For this review, take the finished solid that the model builds, in its own axes (mm). Face numbers are marked on the shaded views. A direction names the side the tool comes from. Round coordinates to 2 decimals unless told otherwise and drop trailing zeros. Write each loop counter-clockwise with the first axis right and the second up, starting at its lowest first coordinate (ties: lowest second). Pieces come first, ordered by that corner, then holes. Notation, with made-up numbers: (78, 83.25) -> (126, 83.25) arc R14 cw to (126, 103.25) -> close; hole circle Ø7 at (29, -8). An arc over 180 degrees is marked (long way). Answer in a Markdown table with one row per item. Add a question column.
```python
from build123d import *

# Parameters (mm, degrees)
SKETCH1_R           = 1.425
BOSS_EXTRUDE1_DEPTH = 4
SKETCH2_W           = 217.15
SKETCH2_H           = 5
BOSS_EXTRUDE2_DEPTH = 24
FILLET1_R           = 4
FILLET2_R           = 3


with BuildPart() as part:
    # Sketch1 → Boss-Extrude1 (new body)
    with BuildSketch(Plane.XY):
        Polygon((110, -15), (90, -15), (90, -5), (-90, -5), (-90, -15), (-107.15, -15), (-107.15, 15), (-90, 15), (-90, 5), (90, 5), (90, 15), (110, 15), align=None)
        with Locations((100, 10)):
            Circle(SKETCH1_R, mode=Mode.SUBTRACT)
        with Locations((100, -10)):
            Circle(SKETCH1_R, mode=Mode.SUBTRACT)
        with Locations((-100, -10)):
            Circle(SKETCH1_R, mode=Mode.SUBTRACT)
        with Locations((-100, 10)):
            Circle(SKETCH1_R, mode=Mode.SUBTRACT)
    extrude(amount=-BOSS_EXTRUDE1_DEPTH)

    # Sketch2 → Boss-Extrude2 (add)
    with BuildSketch(Plane(origin=(0, 0, -4), x_dir=(-1, 0, 0), z_dir=(0, 0, -1))):
        with Locations((-1.425, 0)):
            Rectangle(SKETCH2_W, SKETCH2_H)
    extrude(amount=BOSS_EXTRUDE2_DEPTH)

    # Fillet1
    # the kernel refuses this fillet: 4 mm, written as the material it adds along each edge
    with BuildSketch(Plane(origin=(-107.15, 2.5, -4), x_dir=(0, 1, 0), z_dir=(1, 0, 0))) as fillet1_piece_1_section:
        with BuildLine():
            CenterArc((FILLET1_R, -FILLET1_R), FILLET1_R, 90, 90)
            Line((0, -FILLET1_R), (0, 0))
            Line((0, 0), (FILLET1_R, 0))
        make_face()
    fillet1_piece_1 = extrude(amount=217.15, mode=Mode.PRIVATE)
    fillet1_piece_1 = split(fillet1_piece_1, bisect_by=Plane(origin=(-98.575, 5, -4.029214959), z_dir=(0, 1, 0)), keep=Keep.TOP, mode=Mode.PRIVATE)
    fillet1_piece_1 = split(fillet1_piece_1, bisect_by=Plane(origin=(-90, 5.544093945, -4.029214959), z_dir=(-1, 0, 0)), keep=Keep.TOP, mode=Mode.PRIVATE)
    add(fillet1_piece_1)
    with BuildSketch(Plane(origin=(-107.15, 2.5, -4), x_dir=(0, 1, 0), z_dir=(1, 0, 0))) as fillet1_piece_2_section:
        with BuildLine():
            CenterArc((FILLET1_R, -FILLET1_R), FILLET1_R, 90, 90)
            Line((0, -FILLET1_R), (0, 0))
            Line((0, 0), (FILLET1_R, 0))
        make_face()
    fillet1_piece_2 = extrude(amount=217.15, mode=Mode.PRIVATE)
    fillet1_piece_2 = split(fillet1_piece_2, bisect_by=Plane(origin=(-98.575, 5, -4.966148005), z_dir=(0, -1, 0)), keep=Keep.TOP, mode=Mode.PRIVATE)
    fillet1_piece_2 = split(fillet1_piece_2, bisect_by=Plane(origin=(-90, 3.257783084, -4.966148005), z_dir=(-1, 0, 0)), keep=Keep.TOP, mode=Mode.PRIVATE)
    add(fillet1_piece_2)
    with BuildSketch(Plane(origin=(-107.15, 2.5, -4), x_dir=(0, 1, 0), z_dir=(1, 0, 0))) as fillet1_piece_3_section:
        with BuildLine():
            CenterArc((FILLET1_R, -FILLET1_R), FILLET1_R, 90, 90)
            Line((0, -FILLET1_R), (0, 0))
            Line((0, 0), (FILLET1_R, 0))
        make_face()
    fillet1_piece_3 = extrude(amount=217.15, mode=Mode.PRIVATE)
    fillet1_piece_3 = split(fillet1_piece_3, bisect_by=Plane(origin=(90, 3.257783084, -4.966148005), z_dir=(-1, 0, 0)), keep=Keep.TOP, mode=Mode.PRIVATE)
    fillet1_piece_3 = split(fillet1_piece_3, bisect_by=Plane(origin=(0, 5, -4.966148005), z_dir=(0, -1, 0)), keep=Keep.TOP, mode=Mode.PRIVATE)
    fillet1_piece_3 = split(fillet1_piece_3, bisect_by=Plane(origin=(-90, 3.257783084, -4.966148005), z_dir=(1, 0, 0)), keep=Keep.TOP, mode=Mode.PRIVATE)
    add(fillet1_piece_3)
    with BuildSketch(Plane(origin=(-107.15, 2.5, -4), x_dir=(0, 1, 0), z_dir=(1, 0, 0))) as fillet1_piece_4_section:
        with BuildLine():
            CenterArc((FILLET1_R, -FILLET1_R), FILLET1_R, 90, 90)
            Line((0, -FILLET1_R), (0, 0))
            Line((0, 0), (FILLET1_R, 0))
        make_face()
    fillet1_piece_4 = extrude(amount=217.15, mode=Mode.PRIVATE)
    fillet1_piece_4 = split(fillet1_piece_4, bisect_by=Plane(origin=(90, 5.544093945, -4.029214959), z_dir=(1, 0, 0)), keep=Keep.TOP, mode=Mode.PRIVATE)
    fillet1_piece_4 = split(fillet1_piece_4, bisect_by=Plane(origin=(100, 5, -4.029214959), z_dir=(0, 1, 0)), keep=Keep.TOP, mode=Mode.PRIVATE)
    add(fillet1_piece_4)
    with BuildSketch(Plane(origin=(-107.15, 2.5, -4), x_dir=(0, 1, 0), z_dir=(1, 0, 0))) as fillet1_piece_5_section:
        with BuildLine():
            CenterArc((FILLET1_R, -FILLET1_R), FILLET1_R, 90, 90)
            Line((0, -FILLET1_R), (0, 0))
            Line((0, 0), (FILLET1_R, 0))
        make_face()
    fillet1_piece_5 = extrude(amount=217.15, mode=Mode.PRIVATE)
    fillet1_piece_5 = split(fillet1_piece_5, bisect_by=Plane(origin=(90, 3.257783084, -4.966148005), z_dir=(1, 0, 0)), keep=Keep.TOP, mode=Mode.PRIVATE)
    fillet1_piece_5 = split(fillet1_piece_5, bisect_by=Plane(origin=(100, 5, -4.966148005), z_dir=(0, -1, 0)), keep=Keep.TOP, mode=Mode.PRIVATE)
    add(fillet1_piece_5)
    with BuildSketch(Plane(origin=(110, -2.5, -4), x_dir=(0, -1, 0), z_dir=(-1, 0, 0))) as fillet1_piece_6_section:
        with BuildLine():
            CenterArc((FILLET1_R, -FILLET1_R), FILLET1_R, 90, 90)
            Line((0, -FILLET1_R), (0, 0))
            Line((0, 0), (FILLET1_R, 0))
        make_face()
    fillet1_piece_6 = extrude(amount=217.15, mode=Mode.PRIVATE)
    fillet1_piece_6 = split(fillet1_piece_6, bisect_by=Plane(origin=(90, -5.544093945, -4.029214959), z_dir=(1, 0, 0)), keep=Keep.TOP, mode=Mode.PRIVATE)
    fillet1_piece_6 = split(fillet1_piece_6, bisect_by=Plane(origin=(100, -5, -4.029214959), z_dir=(0, -1, 0)), keep=Keep.TOP, mode=Mode.PRIVATE)
    add(fillet1_piece_6)
    with BuildSketch(Plane(origin=(110, -2.5, -4), x_dir=(0, -1, 0), z_dir=(-1, 0, 0))) as fillet1_piece_7_section:
        with BuildLine():
            CenterArc((FILLET1_R, -FILLET1_R), FILLET1_R, 90, 90)
            Line((0, -FILLET1_R), (0, 0))
            Line((0, 0), (FILLET1_R, 0))
        make_face()
    fillet1_piece_7 = extrude(amount=217.15, mode=Mode.PRIVATE)
    fillet1_piece_7 = split(fillet1_piece_7, bisect_by=Plane(origin=(90, -3.257783084, -4.966148005), z_dir=(1, 0, 0)), keep=Keep.TOP, mode=Mode.PRIVATE)
    fillet1_piece_7 = split(fillet1_piece_7, bisect_by=Plane(origin=(100, -5, -4.966148005), z_dir=(0, 1, 0)), keep=Keep.TOP, mode=Mode.PRIVATE)
    add(fillet1_piece_7)
    with BuildSketch(Plane(origin=(110, -2.5, -4), x_dir=(0, -1, 0), z_dir=(-1, 0, 0))) as fillet1_piece_8_section:
        with BuildLine():
            CenterArc((FILLET1_R, -FILLET1_R), FILLET1_R, 90, 90)
            Line((0, -FILLET1_R), (0, 0))
            Line((0, 0), (FILLET1_R, 0))
        make_face()
    fillet1_piece_8 = extrude(amount=217.15, mode=Mode.PRIVATE)
    fillet1_piece_8 = split(fillet1_piece_8, bisect_by=Plane(origin=(90, -3.257783084, -4.966148005), z_dir=(-1, 0, 0)), keep=Keep.TOP, mode=Mode.PRIVATE)
    fillet1_piece_8 = split(fillet1_piece_8, bisect_by=Plane(origin=(-90, -3.257783084, -4.966148005), z_dir=(1, 0, 0)), keep=Keep.TOP, mode=Mode.PRIVATE)
    fillet1_piece_8 = split(fillet1_piece_8, bisect_by=Plane(origin=(0, -5, -4.966148005), z_dir=(0, 1, 0)), keep=Keep.TOP, mode=Mode.PRIVATE)
    add(fillet1_piece_8)
    with BuildSketch(Plane(origin=(110, -2.5, -4), x_dir=(0, -1, 0), z_dir=(-1, 0, 0))) as fillet1_piece_9_section:
        with BuildLine():
            CenterArc((FILLET1_R, -FILLET1_R), FILLET1_R, 90, 90)
            Line((0, -FILLET1_R), (0, 0))
            Line((0, 0), (FILLET1_R, 0))
        make_face()
    fillet1_piece_9 = extrude(amount=217.15, mode=Mode.PRIVATE)
    fillet1_piece_9 = split(fillet1_piece_9, bisect_by=Plane(origin=(-90, -5.544093945, -4.029214959), z_dir=(-1, 0, 0)), keep=Keep.TOP, mode=Mode.PRIVATE)
    fillet1_piece_9 = split(fillet1_piece_9, bisect_by=Plane(origin=(-98.575, -5, -4.029214959), z_dir=(0, -1, 0)), keep=Keep.TOP, mode=Mode.PRIVATE)
    add(fillet1_piece_9)
    with BuildSketch(Plane(origin=(110, -2.5, -4), x_dir=(0, -1, 0), z_dir=(-1, 0, 0))) as fillet1_piece_10_section:
        with BuildLine():
            CenterArc((FILLET1_R, -FILLET1_R), FILLET1_R, 90, 90)
            Line((0, -FILLET1_R), (0, 0))
            Line((0, 0), (FILLET1_R, 0))
        make_face()
    fillet1_piece_10 = extrude(amount=217.15, mode=Mode.PRIVATE)
    fillet1_piece_10 = split(fillet1_piece_10, bisect_by=Plane(origin=(-90, -3.257783084, -4.966148005), z_dir=(-1, 0, 0)), keep=Keep.TOP, mode=Mode.PRIVATE)
    fillet1_piece_10 = split(fillet1_piece_10, bisect_by=Plane(origin=(-98.575, -5, -4.966148005), z_dir=(0, 1, 0)), keep=Keep.TOP, mode=Mode.PRIVATE)
    add(fillet1_piece_10)

    # Fillet2
    # the kernel refuses this fillet: 3 mm, written as the material it takes off along each edge
    with BuildSketch(Plane(origin=(117.5, -2.5, -28), x_dir=(0, 1, 0), z_dir=(-1, 0, 0))) as fillet2_piece_1:
        with BuildLine():
            CenterArc((FILLET2_R, -FILLET2_R), FILLET2_R, 90, 90)
            Line((0, -FILLET2_R), (0, 0))
            Line((0, 0), (FILLET2_R, 0))
        make_face()
    extrude(amount=232.15, mode=Mode.SUBTRACT)
    with BuildSketch(Plane(origin=(-114.65, 2.5, -28), x_dir=(0, 0, 1), z_dir=(1, 0, 0))) as fillet2_piece_2:
        with BuildLine():
            CenterArc((FILLET2_R, FILLET2_R), FILLET2_R, 180, 90)
            Line((0, FILLET2_R), (0, 0))
            Line((0, 0), (FILLET2_R, 0))
        make_face()
    extrude(amount=232.15, mode=Mode.SUBTRACT)


solid = part.part
```
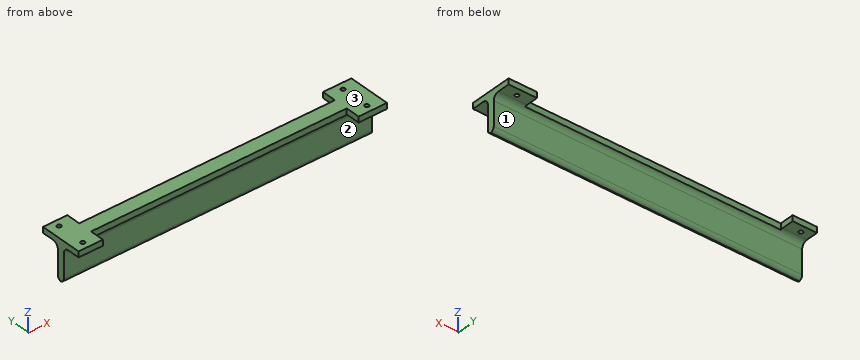
1. We need section B-B (z = -18.5). Write out the cut boundary in (x, y).
2. Clearance check with flat-ended pins moving along their axes: pin 1 Ø2.5 at (x, y) = (-100, -10) entering from +Z; pin 2 Ø2.5 at (x, y) = (-94.5, 8.5) entering from -Z; pin 3 Ø1 at (x, z) = (32.5, -9.5) entering from -Y; pin 4 Ø1.3 at (x, z) = (34, -2.5) entering from +Y. State where each tip first meets the part, or that it passes through.
3. We need section A-A (x = 72.5). Write out the cut boundary in (y, z), plus the area to 3 significant figures.
4. Tool access review of the marked faces 1, 2 and 3: name each direction out of +Z, -Z, +X, -X, +Y, -Y from which nothing blocks a thin tool from reaching the whole face with its end or side.
5. For L1, parallel to Y at x = 100, z = -2.35 (3 decimals); L2, parallel to X at y = 8.5, z = -1.25; L3, parallel to Y at x = -13, z = -3.25, list the stretches that pass through material, from the lowest coordinate up. Write a range as [from, to].
Response:
| question | item | result |
|---|---|---|
| 1 | outline | (-107.15, -2.5) -> (110, -2.5) -> (110, 2.5) -> (-107.15, 2.5) -> close |
| 2 | pin 1 | through |
| 2 | pin 2 | z = -4 |
| 2 | pin 3 | y = -2.5 |
| 2 | pin 4 | y = 5 |
| 3 | outline | (-5, -4.29) arc R4 cw to (-2.5, -8) -> (-2.5, -25) arc R3 ccw to (0, -27.96) arc R3 ccw to (2.5, -25) -> (2.5, -8) arc R4 cw to (5, -4.29) -> (5, 0) -> (-5, 0) -> close |
| 3 | area | 163 mm2 |
| 4 | face 1 | -Z, +X, -X, +Y |
| 4 | face 2 | -Z, +X, -X, -Y |
| 4 | face 3 | +Z, +X, -X, +Y, -Y |
| 5 | L1 | [-15, -11.425], [-8.575, 8.575], [11.425, 15] |
| 5 | L2 | [-107.15, -90], [90, 110] |
| 5 | L3 | [-5, 5] |
